```python
from build123d import *

# Parameters (mm, degrees)
SKETCH_W             = 25
SKETCH_H             = 37
PAD_DEPTH            = 1.5
SKETCH001_W          = 16
SKETCH001_H          = 26
PAD001_DEPTH         = 8.5
SKETCH002_W          = 18
SKETCH002_H          = 32.5
PAD002_DEPTH         = 9
SKETCH003_W          = 8
SKETCH003_H          = 2.5
PAD003_DEPTH         = 2
BODY_PITCH_ANGLE     = 90
BODY_PLACEMENT_ANGLE = -90


with BuildPart() as part:
    # Sketch → Pad (new body)
    with BuildSketch(Plane.YZ):
        with Locations((4.273874, -1.909899)):
            Rectangle(SKETCH_W, SKETCH_H)
    extrude(amount=PAD_DEPTH)

    # Sketch001 (on Face5 of Pad) → Pad001 (join)
    with BuildSketch(Plane(origin=(0, 0, 0), x_dir=(0, 1, 0), z_dir=(-1, 0, 0))):
        with Locations((3.273874, 5.909899)):
            Rectangle(SKETCH001_W, SKETCH001_H)
    extrude(amount=PAD001_DEPTH)

    # Sketch002 (on Face5 of Pad001) → Pad002 (join)
    with BuildSketch(Plane.YZ.offset(1.5)):
        with Locations((2.773874, -2.159899)):
            Rectangle(SKETCH002_W, SKETCH002_H)
    extrude(amount=PAD002_DEPTH)

    # Sketch003 (on Face14 of Pad002) → Pad003 (join)
    with BuildSketch(Plane(origin=(0, 0, 14.090101), x_dir=(0, -1, 0), z_dir=(0, 0, 1))):
        with Locations((-2.773874, 6.25)):
            Rectangle(SKETCH003_W, SKETCH003_H)
    extrude(amount=PAD003_DEPTH)


with BuildPart() as part_1:
    # Body pitch: moved
    add(part.part.rotate(Axis((0, 0, 0), (0, 1, 0)), BODY_PITCH_ANGLE))


with BuildPart() as part_2:
    # Body placement: moved
    add(part_1.part.moved(Location((7.68397, -0.0001, 3.86387))).rotate(Axis((7.68397, -0.0001, 3.86387), (0, 0, 1)), BODY_PLACEMENT_ANGLE))


solid = part_2.part
```
The model under review builds one solid part; all positions refer to its coordinate system, in mm. A direction names the side the tool comes from. Round coordinates to 2 decimals unless told otherwise and drop trailing zeros. Order: outer loops, then holes, each group sorted by start corner. A loop starts at its lowest first (then second) coordinate and runs counter-clockwise, first axis right, second up. Notation, with made-up numbers: (50, 17.5) -> (75, 17.5) arc R10 ccw to (75, 25.5) -> close; hole circle Ø7 at (22.5, 37.5). An arc over 180 degrees is marked (long way). One line per item, written item: value. Start each with the question number.
Q1. Take a section at D-D (x = 15.75). Write out the cut boundary in (y, z).
Q2. Mouldability with a two-part tool opening along Z and no side actions: class faces 1 (the face through (18.958, 6, 8)), 2 (the face through (11, 6, 12.364)), 3 (the face through (10, -14.09, 0)) as released by +Z, released by -Z, zero draft, split by the parting line, or undercut.
Q3. Machinability: for faces 4 (the face through (6.458, -15, -2)), 5 (the face through (11, -7.09, 8)), 6 (the face through (19.458, 2, -2)), which of the approach directions +Z, -Z, +X, -X, +Y, -Y give a long, thin tool a straight path to every point of the face, cutting with its end or side? Answer none if there is none.
Q4. Clearance check with flat-ended pins moving along their axes: pin 1 Ø4.5 at (x, z) = (9, 0) entering from -Y; pin 2 Ø4.5 at (y, z) = (0.5, 9.5) entering from -X; pin 3 Ø2.5 at (y, z) = (7.5, 9.5) entering from +X. State where each tip first meets the part, or that it passes through.
Q5. Take a section at C-C (z = -2.75). Write out the cut boundary in (x, y), and give its area (3 significant figures).
Q6. Wall thickness on line 1 (Y direction, x = 14.25, z = -4.75); line 2 (X direction, y = 4, z = 8.25); line 3 (X direction, y = -11.5, z = 0.5): over which ranges is each line inside the solid? List them lowest first.
Q7. Take a section at A-A (y = -13). Write out the cut boundary in (x, z).
Q8. Take a section at B-B (x = 12.25). Write out the cut boundary in (y, z), and give its area (3 significant figures).
Reported:
1. outline: (-16.59, 2.36) -> (-14.09, 2.36) -> (-14.09, -6.64) -> (18.41, -6.64) -> (18.41, 2.36) -> (20.41, 2.36) -> (20.41, 3.86) -> (18.91, 3.86) -> (18.91, 12.36) -> (-7.09, 12.36) -> (-7.09, 3.86) -> (-16.59, 3.86) -> close
2. face 1: zero draft
2. face 2: released by +Z
2. face 3: undercut
3. face 4: -Z, -X, -Y
3. face 5: +Z, +X, -X, -Y
3. face 6: -Z, +X, +Y, -Y
4. pin 1: stops at y = -16.09
4. pin 2: stops at x = 2.96
4. pin 3: stops at x = 18.96
5. outline: (1.46, -14.09) -> (6.46, -14.09) -> (6.46, -16.09) -> (14.46, -16.09) -> (14.46, -14.09) -> (19.46, -14.09) -> (19.46, 18.41) -> (1.46, 18.41) -> close
5. area: 601 mm2
6. line 1: y = -14.09 to 18.41
6. line 2: x = 2.96 to 18.96
6. line 3: x = 1.46 to 19.46
7. outline: (-0.54, 2.36) -> (1.46, 2.36) -> (1.46, -6.64) -> (19.46, -6.64) -> (19.46, 2.36) -> (24.46, 2.36) -> (24.46, 3.86) -> (-0.54, 3.86) -> close
8. outline: (-16.59, 2.36) -> (-14.09, 2.36) -> (-14.09, -1.14) -> (-16.09, -1.14) -> (-16.09, -3.64) -> (-14.09, -3.64) -> (-14.09, -6.64) -> (18.41, -6.64) -> (18.41, 2.36) -> (20.41, 2.36) -> (20.41, 3.86) -> (18.91, 3.86) -> (18.91, 12.36) -> (-7.09, 12.36) -> (-7.09, 3.86) -> (-16.59, 3.86) -> close
8. area: 574 mm2
